Build history of the part. All positions in model axes, mm. Face numbers are marked on the shaded views. Coordinates: 2 decimals unless noted, no trailing zeros. Order: outer loops, then holes, each group sorted by start corner. A loop starts at its lowest first (then second) coordinate and runs counter-clockwise, first axis right, second up. Notation, with made-up numbers: (-31.75, 19.5) - (12.25, 19.5) arc R23 ccw to (12.25, 52.5) - close; hole circle Ø11 at (65.25, 85.5). An arc over 180 degrees is marked (long way). Write each question's results on one line, items separated by ' | '.
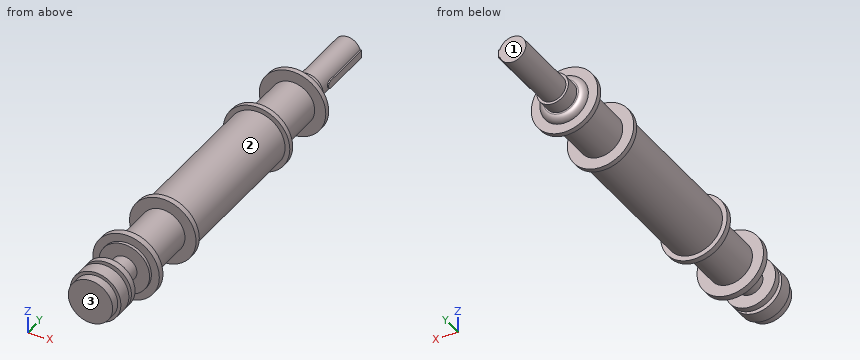
from build123d import *

# Parameters (mm, degrees)
F0_R      = 21
F1_DEPTH  = 110
F3_DEPTH  = 22.5
F4_R      = 25
F5_DEPTH  = 23
F6_R      = 37.5
F7_DEPTH  = 10
F8_R      = 9.99999
F9_R      = 52.5
F9_R_2    = 37.5
F10_DEPTH = 8
F11_R     = 35
F12_DEPTH = 91
F13_R     = 52.5
F14_DEPTH = 8
F15_R     = 45
F16_DEPTH = 249
F17_R     = 52.5
F18_DEPTH = 9
F19_R     = 35
F20_DEPTH = 91
F21_R     = 52.5
F22_DEPTH = 10
F23_R     = 40
F24_DEPTH = 5
F25_R     = 20
F26_DEPTH = 40
F27_R     = 40
F28_DEPTH = 10
F29_R     = 30
F30_DEPTH = 7
F31_R     = 40
F32_DEPTH = 22
F33_R     = 35
F34_DEPTH = 14


# Not quite as in the source:
# - a fillet or chamfer is up to 0.001 mm smaller than in the source, because OpenCascade refuses the exact size


with BuildPart() as f1:
    # F0 (on Front) → F1 (new body)
    with BuildSketch(Plane.XZ):
        Circle(F0_R)
    extrude(amount=F1_DEPTH)

    # F2 (on Right) → F3 (join)
    with BuildSketch(Plane.YZ):
        with BuildLine():
            Line((0, -6), (0, 6))
            Line((0, 6), (-85, 6))
            ThreePointArc((-85, 6), (-91, 0), (-85, -6))
            Line((-85, -6), (0, -6))
        make_face()
    extrude(amount=F3_DEPTH)

    # F4 (on face) → F5 (join)
    with BuildSketch(Plane.XZ.offset(110)):
        Circle(F4_R)
    extrude(amount=F5_DEPTH)

    # F6 (on face) → F7 (join)
    with BuildSketch(Plane.XZ.offset(133)):
        Circle(F6_R)
    extrude(amount=F7_DEPTH)

    # F8 (radius 10 in the source; OpenCascade refuses exactly that, so slightly less here)
    f8_edges = [f1.edges().sort_by_distance(p)[0] for p in [
        (-37.5, -133, 0),
    ]]
    fillet(f8_edges, radius=F8_R)

    # F9 (on face) → F10 (join)
    with BuildSketch(Plane.XZ.offset(143)):
        Circle(F9_R)
        Circle(F9_R_2, mode=Mode.SUBTRACT)
        Circle(F9_R_2)
    extrude(amount=F10_DEPTH)

    # F11 (on face) → F12 (join)
    with BuildSketch(Plane.XZ.offset(151)):
        Circle(F11_R)
    extrude(amount=F12_DEPTH)

    # F13 (on face) → F14 (join)
    with BuildSketch(Plane.XZ.offset(242)):
        Circle(F13_R)
    extrude(amount=F14_DEPTH)

    # F15 (on face) → F16 (join)
    with BuildSketch(Plane.XZ.offset(250)):
        Circle(F15_R)
    extrude(amount=F16_DEPTH)

    # F17 (on face) → F18 (join)
    with BuildSketch(Plane.XZ.offset(499)):
        Circle(F17_R)
    extrude(amount=F18_DEPTH)

    # F19 (on face) → F20 (join)
    with BuildSketch(Plane.XZ.offset(508)):
        Circle(F19_R)
    extrude(amount=F20_DEPTH)

    # F21 (on face) → F22 (join)
    with BuildSketch(Plane.XZ.offset(599)):
        Circle(F21_R)
    extrude(amount=F22_DEPTH)

    # F23 (on face) → F24 (join)
    with BuildSketch(Plane.XZ.offset(609)):
        Circle(F23_R)
    extrude(amount=F24_DEPTH)

    # F25 (on face) → F26 (join)
    with BuildSketch(Plane.XZ.offset(614)):
        Circle(F25_R)
    extrude(amount=F26_DEPTH)

    # F27 (on face) → F28 (join)
    with BuildSketch(Plane.XZ.offset(654)):
        Circle(F27_R)
    extrude(amount=F28_DEPTH)

    # F29 (on face) → F30 (join)
    with BuildSketch(Plane.XZ.offset(664)):
        Circle(F29_R)
    extrude(amount=F30_DEPTH)

    # F31 (on face) → F32 (join)
    with BuildSketch(Plane.XZ.offset(671)):
        Circle(F31_R)
    extrude(amount=F32_DEPTH)

    # F33 (on face) → F34 (join)
    with BuildSketch(Plane.XZ.offset(693)):
        Circle(F33_R)
    extrude(amount=F34_DEPTH)


solid = f1.part
1. Band-saw the part on B-B on y = -330.5. Give the cut face in (x, z).
Solved:
outline: circle Ø90 at (0, 0)
2. Band-saw the part on A-A on y = -167. Give the cut face in (x, z).
Solved:
outline: circle Ø70 at (0, 0)
3. Drop flat-ended pins along their axis: pin 1 Ø9.5 at (y, z) = (-29, 2.5) entering from +X; pin 2 Ø6 at (x, y) = (25, -568.5) entering from -Z; pin 3 Ø10 at (x, y) = (39, -425.5) entering from -Z. Give the stop position or say it passes through.
Solved:
pin 1: stops at x = 22.5 | pin 2: stops at z = -27.22 | pin 3: stops at z = -29.48
4. Two-plate mould, pull along Y, no slides. Class the marked faces 1, 2 and 3: +Y half, -Y half, draft (parallel to the pull), parting line (faces both ways), or undercut.
Solved:
face 1: +Y half | face 2: undercut | face 3: -Y half
5. Probe line 1 (Y direction, x = 22, z = -45); line 2 (Y direction, x = 5, z = 40.5); line 3 (Y direction, x = 38.5, z = -2.5). List the from-to ranges inside material, lowest first.
Solved:
line 1: y = -609 to -599, -508 to -499, -250 to -242, -151 to -143 | line 2: y = -609 to -599, -508 to -242, -151 to -143 | line 3: y = -693 to -671, -664 to -654, -614 to -599, -508 to -242, -151 to -143
